from build123d import *

# Parameters (mm, degrees)
SKETCH1_R           = 2
BOSS_EXTRUDE1_DEPTH = 1
SKETCH2_R           = 1
CUT_EXTRUDE1_DEPTH  = 16.244753196
FILLET1_R           = 0.75
CHAMFER1_SIZE       = 0.4
SKETCH3_R           = 0.4572
CUT_EXTRUDE2_DEPTH  = 16.244753196


with BuildPart() as part:
    # Sketch1 → Boss-Extrude1 (new body)
    with BuildSketch(Plane(origin=(0, 0, 0), x_dir=(1, 0, 0), z_dir=(0, 1, 0))):
        Polygon((12, 5.95), (-3.9, 5.95), (-3.9, -5.95), (12, -5.95), (12, -4.025), (14, -4.025), (14, 4.025), (12, 4.025), align=None)
        with Locations(Location((0, 0, 0), (0, 0, 270))):
            Circle(SKETCH1_R, mode=Mode.SUBTRACT)
    extrude(amount=BOSS_EXTRUDE1_DEPTH)

    # Sketch2 → Cut-Extrude1 (cut, through all)
    with BuildSketch(Plane(origin=(0, 1, 0), x_dir=(1, 0, 0), z_dir=(0, 1, 0))):
        with Locations(Location((-2.35, 4.25, 0), (0, 0, 270))):
            Circle(SKETCH2_R)
        with Locations(Location((-2.35, -4.25, 0), (0, 0, 270))):
            Circle(SKETCH2_R)
    extrude(amount=-CUT_EXTRUDE1_DEPTH, mode=Mode.SUBTRACT)

    # Fillet1
    fillet1_edges = [part.edges().sort_by_distance(p)[0] for p in [
        (-3.9, 0.5, -5.95),
        (-3.9, 0.5, 5.95),
    ]]
    fillet(fillet1_edges, radius=FILLET1_R)

    # Chamfer1
    chamfer1_edges = [part.edges().sort_by_distance(p)[0] for p in [
        (-2.35, 0, -5.25),
        (-2.35, 0, 3.25),
    ]]
    chamfer(chamfer1_edges, length=CHAMFER1_SIZE)

    # Sketch3 → Cut-Extrude2 (cut, through all)
    with BuildSketch(Plane(origin=(0, 1, 0), x_dir=(1, 0, 0), z_dir=(0, 1, 0))):
        with Locations(Location((3.61862915, -3.1, 0), (0, 0, 270))):
            Circle(SKETCH3_R)
        with Locations(Location((4.75, 0, 0), (0, 0, 270))):
            Circle(SKETCH3_R)
        with Locations(Location((6.247772136, 2.94052353, 0), (0, 0, 270))):
            Circle(SKETCH3_R)
        with Locations(Location((9.5, 3.5, 0), (0, 0, 270))):
            Circle(SKETCH3_R)
    extrude(amount=-CUT_EXTRUDE2_DEPTH, mode=Mode.SUBTRACT)

    # Sketch5 → CSK for M1.6 Countersunk Raised Head Screw2 (revolve, cut)
    with BuildSketch(Plane(origin=(12.5, 0, 0), x_dir=(0, 0, -1), z_dir=(1, 0, 0))):
        Polygon((0, 0), (0, 1), (0.85, 1), (0.85, 0.55), (1.4, 0), align=None)
    revolve(axis=Axis((12.5, -6.35, 0), (0, 1, 0)), mode=Mode.SUBTRACT)


solid = part.part
Check sheet for the modelled part. Datum: model origin and axes. Units: mm. A direction names the side the tool comes from. Give positions to 0.01 mm unless a question says otherwise; leave off trailing zeros. Write each loop counter-clockwise with the first axis right and the second up, starting at its lowest first coordinate (ties: lowest second). Pieces come first, ordered by that corner, then holes. Notation, with made-up numbers: (11, -3.5) -> (63, -3.5) arc R13 cw to (63, 12.5) -> close; hole circle Ø9 at (1, 41.25). An arc over 180 degrees is marked (long way). Write item = value, one per line.
Item 1: Sectioned sample at D-D on z = 0. Record the boundary of the cut face in (x, y), and give its area (3 significant figures).
Output:
outline = (-3.9, 0) -> (-2, 0) -> (-2, 1) -> (-3.9, 1) -> close; (2, 0) -> (4.29, 0) -> (4.29, 1) -> (2, 1) -> close; (5.21, 0) -> (11.1, 0) -> (11.65, 0.55) -> (11.65, 1) -> (5.21, 1) -> close; (13.35, 0.55) -> (13.9, 0) -> (14, 0) -> (14, 1) -> (13.35, 1) -> close
area = 11.0 mm^2
Item 2: Scan lines: probe 1 along X at (y, z) = (0.3, 0); probe 2 along X at (y, z) = (0.65, -3.5); probe 3 along Z at (x, y) = (-1.75, 0.95). Record each from-to range of solid material in increasing order. Write a range as from..to.
Output:
probe_1 = -3.9..-2, 2..4.29, 5.21..11.4, 13.6..14
probe_2 = -3.9..-3.01, -1.69..9.04, 9.96..14
probe_3 = -5.95..-5.05, -3.45..-0.97, 0.97..3.45, 5.05..5.95
Item 3: Sectioned sample at B-B on z = 4.25. Record the boundary of the cut face in (x, y), and give its area (3 significant figures).
Output:
outline = (-3.9, 0) -> (-3.75, 0) -> (-3.35, 0.4) -> (-3.35, 1) -> (-3.9, 1) -> close; (-1.35, 0.4) -> (-0.95, 0) -> (12, 0) -> (12, 1) -> (-1.35, 1) -> close
area = 13.7 mm^2
Item 4: Sectioned sample at A-A on x = 9.5. Record the boundary of the cut face in (y, z), and give its area (3 significant figures).
Output:
outline = (0, -5.95) -> (1, -5.95) -> (1, -3.96) -> (0, -3.96) -> close; (0, -3.04) -> (1, -3.04) -> (1, 5.95) -> (0, 5.95) -> close
area = 11.0 mm^2
Item 5: Sectioned sample at C-C on x = -2.35. Record the boundary of the cut face in (y, z), and give its area (3 significant figures).
Output:
outline = (0, -5.95) -> (1, -5.95) -> (1, -5.25) -> (0.4, -5.25) -> (0, -5.65) -> close; (0, -2.85) -> (0.4, -3.25) -> (1, -3.25) -> (1, 3.25) -> (0.4, 3.25) -> (0, 2.85) -> close; (0, 5.65) -> (0.4, 5.25) -> (1, 5.25) -> (1, 5.95) -> (0, 5.95) -> close
area = 7.58 mm^2
Item 6: Tool access check on faces 1 (the cylindrical face through (-2.96, 0.7, -5.04)), 2 (the flat face through (13, 0.5, -4.025)), 3 (the flat face through (13, 0.5, 4.025)). Record the directions out of +Z, -Z, +X, -X, +Y, -Y that give a thin tool (end or side, any length) a straight path to the whole face; none if there is none.
Output:
face_1 = +Y, -Y
face_2 = -Z, +X, +Y, -Y
face_3 = +Z, +X, +Y, -Y
Item 7: Gauge pin test, flat ends, axial feed: pin 1 (6.5 mm diameter, centred on x = 0, z = 0, fed in from -Y); pin 2 (2.5 mm diameter, centred on x = 12.5, z = 0, fed in from -Y). Record the tip position at first contact, or that the pin passes through.
Output:
pin_1 = 0
pin_2 = 0.15
